Design review of the part shown in the three views and the two pictorial views. Dimensions are in mm from the part's minimum x, y and z. A direction names the side the tool comes from. Coordinates: 2 decimals unless noted, no trailing zeros. Write each loop counter-clockwise with the first axis right and the second up, starting at its lowest first coordinate (ties: lowest second). Pieces come first, ordered by that corner, then holes. Notation, with made-up numbers: (9, 29.25) - (32, 29.25) arc R28 cw to (32, 52.25) - close; hole circle Ø2 at (58, 84). An arc over 180 degrees is marked (long way). Return JSON: item names as keys, results as strings. Group by question number.
(1) Tool access review of the marked faces 1, 2, 3, 4 and 5: name each direction out of +Z, -Z, +X, -X, +Y, -Y from which nothing blocks a thin tool from reaching the whole face with its end or side.
(2) We need section C-C on y = 3. State the section outline as (x, z) points (1 decimal), then the cut area to 3 significant figures.
(3) For pin 1 Ø3 at (y, z) = (1.5, 3.5) entering from +X; pin 2 Ø3 at (x, y) = (4.5, 3.5) entering from -Z; pin 3 Ø3 at (y, z) = (2.5, 9) entering from -X; pin 4 Ø1.9 at (y, z) = (2.5, 30.5) entering from -X, all flat-tipped, find the tip position at first contact; note any pin that passes through.
(4) We need section D-D on x = 57. State the section outline as (y, z) points.
(5) We need section B-B on z = 31. Give the number of separate pieces and of enclosed holes in the cut face, then the cut area to 3 significant figures.
(6) To check wall thickness, follow L1, parallel to X at y = 3.5, z = 20.4 (1 decimal); L2, parallel to X at y = 3, z = 15.5; L3, parallel to Z at x = 18, y = 2. State the ranges of each line that lie inside material, in increasing order. Write a range as from..to.
(7) We need section A-A on z = 17.5. State the section outline as (x, y) points.
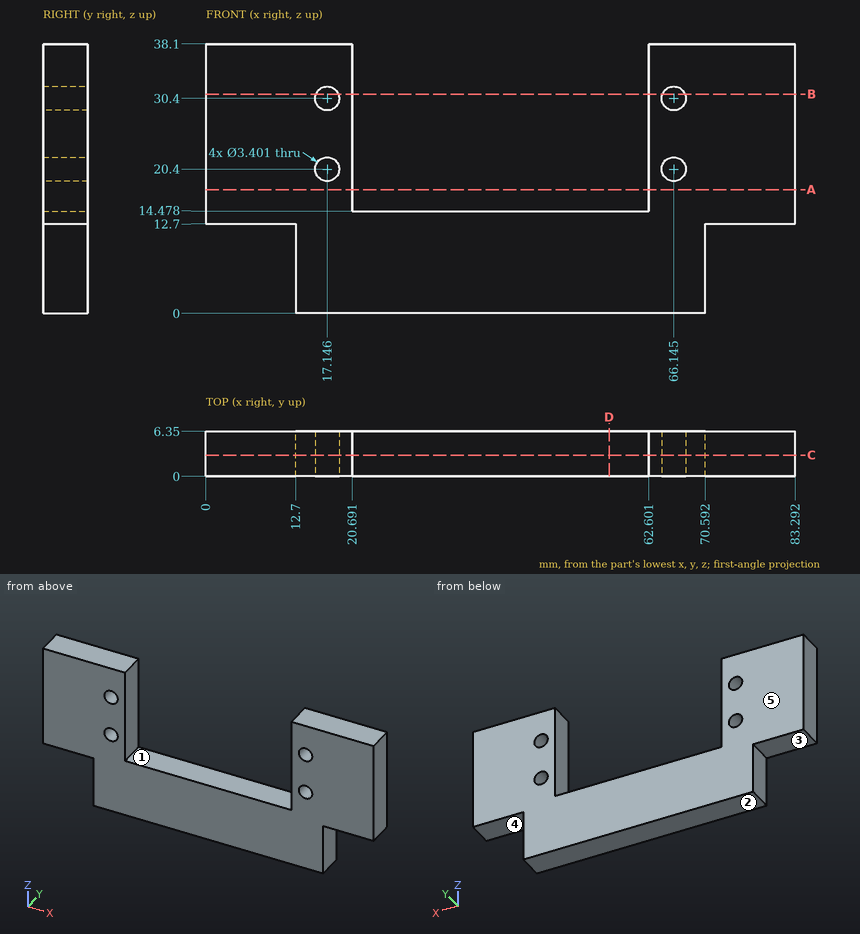
Ans:
{
 "1": {"face 1": "+Z, +Y, -Y", "face 2": "-Z, +X, -X, +Y, -Y", "face 3": "-Z, -X, +Y, -Y", "face 4": "-Z, +X, +Y, -Y", "face 5": "+Z, -Z, +X, -X, +Y"},
 "2": {"outline": "(0, 12.7) - (12.7, 12.7) - (12.7, 0) - (70.6, 0) - (70.6, 12.7) - (83.3, 12.7) - (83.3, 38.1) - (62.6, 38.1) - (62.6, 14.5) - (20.7, 14.5) - (20.7, 38.1) - (0, 38.1) - close; hole circle Ø3.4 at (17.1, 20.4); hole circle Ø3.4 at (17.1, 30.4); hole circle Ø3.4 at (66.1, 20.4); hole circle Ø3.4 at (66.1, 30.4)", "area": "1,820 mm²"},
 "3": {"pin 1": "x = 70.59", "pin 2": "z = 12.7", "pin 3": "x = 12.7", "pin 4": "x = 0"},
 "4": {"outline": "(0, 0) - (6.35, 0) - (6.35, 14.48) - (0, 14.48) - close"},
 "5": {"separate pieces": "4", "enclosed holes": "0", "area": "222 mm²"},
 "6": {"L1": "0..15.4, 18.8..20.7, 62.6..64.4, 67.8..83.3", "L2": "0..20.69, 62.6..83.29", "L3": "0..18.93, 21.87..28.93, 31.87..38.1"},
 "7": {"outline": "(0, 0) - (20.69, 0) - (20.69, 6.35) - (0, 6.35) - close; (62.6, 0) - (83.29, 0) - (83.29, 6.35) - (62.6, 6.35) - close"}
}
